Autodesk Inventor part; units mm, degrees
ref_plane "YZ Plane" through (0, 0, 0) normal (1, 0, 0) x (0, 1, 0)
ref_plane "XZ Plane" through (0, 0, 0) normal (0, 1, 0) x (-1, 0, 0)
ref_plane "XY Plane" through (0, 0, 0) normal (0, 0, 1) x (1, 0, 0)
sketch "Sketch1" plane through (0, 0, 0) normal (0, 0, 1) x (1, 0, 0)
  circle A0 centre (0, 0) radius 5
  arc A1 (-13, 15) -> (-15, 13) centre (-13, 13) ccw
  arc A2 (-15, -13) -> (-13, -15) centre (-13, -13) ccw
  arc A3 (13, -15) -> (15, -13) centre (13, -13) ccw
  arc A4 (15, 13) -> (13, 15) centre (13, 13) ccw
  arc A5 (-13, 14) -> (-14, 13) centre (-13, 13) ccw
  arc A6 (-14, -13) -> (-13, -14) centre (-13, -13) ccw
  arc A7 (13, -14) -> (14, -13) centre (13, -13) ccw
  arc A8 (14, 13) -> (13, 14) centre (13, 13) ccw
  line L0 (14, -14) -> (-14, 14) construction
  line L1 (-14, -14) -> (14, 14) construction
  line L2 (15, -15) -> (-15, 15) construction
  line L3 (-15, -15) -> (15, 15) construction
  line L4 (-13, 15) -> (-8, 15)
  line L5 (-8, 13) -> (-8, 8) construction
  line L6 (-9.4142, 8) -> (-13, 8)
  line L7 (-15, 8) -> (-15, 13)
  line L8 (-13, -15) -> (-8, -15)
  line L9 (-8, -13) -> (-8, -9.4142)
  line L10 (-9.4142, -8) -> (-13, -8)
  line L11 (-15, -8) -> (-15, -13)
  line L12 (13, -15) -> (8, -15)
  line L13 (8, -13) -> (8, -9.4142)
  line L14 (9.4142, -8) -> (13, -8)
  line L15 (15, -8) -> (15, -13)
  line L16 (13, 15) -> (8, 15)
  line L17 (8, 13) -> (8, 9.4142)
  line L18 (9.4142, 8) -> (13, 8)
  line L19 (15, 8) -> (15, 13)
  line L20 (-13, 9) -> (-10, 9)
  line L21 (-9, 10) -> (-9, 13)
  line L22 (-10, 14) -> (-13, 14)
  line L23 (-14, 13) -> (-14, 10)
  line L24 (13, 9) -> (10, 9)
  line L25 (9, 10) -> (9, 13)
  line L26 (10, 14) -> (13, 14)
  line L27 (14, 13) -> (14, 10)
  line L28 (13, -9) -> (10, -9)
  line L29 (9, -10) -> (9, -13)
  line L30 (10, -14) -> (13, -14)
  line L31 (14, -13) -> (14, -10)
  line L32 (-13, -9) -> (-10, -9)
  line L33 (-9, -10) -> (-9, -13)
  line L34 (-10, -14) -> (-13, -14)
  line L35 (-14, -13) -> (-14, -10)
  line L36 (-14, 13) -> (-14, 10)
  line L37 (-14, -10) -> (-14, -13)
  line L38 (-14, -13) -> (-14, -10)
  line L39 (-14, 10) -> (-14, 13)
  line L40 (13, -15) -> (5, -15)
  line L41 (-5, -15) -> (-13, -15)
  line L42 (13, -15) -> (5, -15) construction
  line L43 (0, -15) -> (-13, -15) construction
  line L44 (4, -13) -> (8, -13)
  line L45 (-8, -13) -> (-4, -13)
  line L46 (10, -9) -> (13, -9)
  line L47 (14, -10) -> (14, -13)
  line L48 (13, -14) -> (10, -14)
  line L49 (9, -13) -> (9, -10)
  line L50 (5, -14) -> (5, -15)
  line L51 (13, -14) -> (10, -14)
  line L52 (5, -14) -> (4, -14)
  line L53 (4, -14) -> (5, -14)
  line L54 (10, -14) -> (13, -14)
  line L55 (-4, -14) -> (-5, -14)
  line L56 (-10, -14) -> (-13, -14)
  line L57 (-13, -14) -> (-10, -14)
  line L58 (-5, -14) -> (-4, -14)
  line L59 (14, -13) -> (14, -10)
  line L60 (14, 10) -> (14, 13)
  line L61 (14, 13) -> (14, 10)
  line L62 (14, -10) -> (14, -13)
  line L63 (-5, -14) -> (-5, -15)
  line L64 (10, 14) -> (13, 14)
  line L65 (13, 14) -> (10, 14)
  line L66 (-10, 14) -> (-13, 14)
  line L67 (-13, 14) -> (-10, 14)
  line L68 (-5, 15) -> (-5, 14)
  line L69 (-13, 15) -> (-5, 15)
  line L70 (5, 15) -> (13, 15)
  line L71 (-15, 15) -> (-5, 15) construction
  line L72 (5, 15) -> (15, 15) construction
  line L73 (5, 15) -> (5, 14)
  line L74 (8, 13) -> (4, 13)
  line L75 (5, 14) -> (4, 14)
  line L76 (-5, 14) -> (-4, 14)
  line L77 (4, 14) -> (5, 14)
  line L78 (-4, 13) -> (-8, 13)
  line L79 (-4, 14) -> (-5, 14)
  line L80 (4, 13) -> (4, 14)
  line L81 (-4, 13) -> (-4, 14)
  line L82 (-4, -14) -> (-4, -13)
  line L83 (4, -14) -> (4, -13)
  line L84 (-8, 9.4142) -> (-4.1919, 5.6061)
  line L85 (8, 9.4142) -> (4.1919, 5.6061)
  line L86 (9.4142, 8) -> (5.6061, 4.1919)
  line L87 (5.6061, -4.1919) -> (9.4142, -8)
  line L88 (4.1919, -5.6061) -> (8, -9.4142)
  line L89 (-4.1919, -5.6061) -> (-8, -9.4142)
  line L90 (-5.6061, -4.1919) -> (-9.4142, -8)
  line L91 (-9.4142, 8) -> (-5.6061, 4.1919)
  arc A9 (4.1919, 5.6061) -> (-4.1919, 5.6061) centre (0, 0) ccw
  arc A10 (5.6061, -4.1919) -> (5.6061, 4.1919) centre (0, 0) ccw
  arc A11 (-5.6061, 4.1919) -> (-5.6061, -4.1919) centre (0, 0) ccw
  arc A12 (-4.1919, -5.6061) -> (4.1919, -5.6061) centre (0, 0) ccw
  line L92 (-8, 13) -> (-8, 9.4142)
  line L93 (-15, -13) -> (-15, -5) construction
  line L94 (-15, -13) -> (-15, -5)
  line L95 (-15, 5) -> (-15, 13)
  line L96 (15, -5) -> (15, -13) construction
  line L97 (15, 13) -> (15, 5)
  line L98 (15, -5) -> (15, -13)
  line L99 (-14, -4) -> (-14, -5)
  line L100 (14, -4) -> (14, -5)
  line L101 (14, 4) -> (14, 5)
  line L102 (-14, 4) -> (-14, 5)
  line L103 (-13, 8) -> (-13, 4)
  line L104 (13, 4) -> (13, 8)
  line L105 (13, -8) -> (13, -4)
  line L106 (-13, -4) -> (-13, -8)
  line L107 (-14, -5) -> (-15, -5)
  line L108 (15, -5) -> (14, -5)
  line L109 (15, 5) -> (14, 5)
  line L110 (-14, 5) -> (-15, 5)
  line L111 (13, 4) -> (14, 4)
  line L112 (-14, 4) -> (-13, 4)
  line L113 (-14, -4) -> (-13, -4)
  line L114 (13, -4) -> (14, -4)
  arc A13 (-13, -9) -> (-14, -10) centre (-13, -10) ccw
  arc A14 (-9, -10) -> (-10, -9) centre (-10, -10) ccw
  arc A15 (-10, -14) -> (-9, -13) centre (-10, -13) ccw
  arc A16 (10, -9) -> (9, -10) centre (10, -10) ccw
  arc A17 (9, -13) -> (10, -14) centre (10, -13) ccw
  arc A18 (14, -10) -> (13, -9) centre (13, -10) ccw
  arc A19 (10, 14) -> (9, 13) centre (10, 13) ccw
  arc A20 (9, 10) -> (10, 9) centre (10, 10) ccw
  arc A21 (13, 9) -> (14, 10) centre (13, 10) ccw
  arc A22 (-9, 13) -> (-10, 14) centre (-10, 13) ccw
  arc A23 (-10, 9) -> (-9, 10) centre (-10, 10) ccw
  arc A24 (-14, 10) -> (-13, 9) centre (-13, 10) ccw
  point P0 (15, -15)
  point P1 (-5.5858, -7)
  dimension "d0" = 30
  dimension "d1" = 30
  dimension "d2" = 10
  dimension "d4" = 2
  dimension "d11" = 28
  dimension "d12" = 7
  dimension "d13" = 7
  dimension "d15" = 1
  dimension "d16" = 1
  dimension "d17" = 1
  dimension "d18" = 1
  dimension "d19" = 5
  dimension "d23" = 30
  dimension "d27" = 1
  dimension "d30" = 3.5858
  dimension "d31" = 2
  dimension "d32" = 16
  dimension "d33" = 8
  dimension "d34" = 6
  dimension "d35" = 5.5858
extrude "Extrusion1" add sketch "Sketch1" along normal mid plane 318
properties part number "trail" material "Aluminum 6061"
Check sheet for the modelled part. Datum: model origin and axes. Units: mm. Give positions to 0.01 mm unless a question says otherwise; leave off trailing zeros. Write each loop counter-clockwise with the first axis right and the second up, starting at its lowest first coordinate (ties: lowest second). Pieces come first, ordered by that corner, then holes. Notation, with made-up numbers: (33, -29.75) -> (75, -29.75) arc R23 cw to (75, 0.25) -> close; hole circle Ø2 at (21.5, -25.5). An arc over 180 degrees is marked (long way). Use one line per item in the form item = value. Start each with the question number.
1. Mould release check, pull along Y, two halves, no side actions. Record for faces 1 (the flat face through (-15, -9, -2)), 2 (the flat face through (9, 15, -2)), 3 (the cylindrical face through (-7, 0, -2)): pulls with the +Y half, pulls with the -Y half, needs draft (parallel to the pull), parting line crosses it, or undercut.
2. Thickness scan on line 1 along X through (y, z) = (-12.5, -56); line 2 along Y through (x, z) = (0, -35); line 3 along Y through (x, z) = (-9.5, 15). Record the ranges inside material, lowest first. Write a range as from..to.
3. Section check A-A (x = 0). Record the cut outline in (y, z).
4. Section check C-C (z = -128.5). Count the separate pieces of the cut face and the enclosed holes in it, and give its area (3 significant figures).
5. Go/stop test with a flat-tipped pin: P1, Ø0.8, axis at y = -13.5, z = -67.5, coming from the +X side. Record where the tip stops, or that it passes through.
Conclusion:
q1.face_1 = needs draft
q1.face_2 = pulls with the +Y half
q1.face_3 = undercut
q2.line_1 = -15..-14, -9..-8, 8..9, 14..15
q2.line_2 = -7..-5, 5..7
q2.line_3 = -15..-13.87, -9.13..-8, 8..9.13, 13.87..15
q3.outline = (-7, -159) -> (-5, -159) -> (-5, 159) -> (-7, 159) -> close; (5, -159) -> (7, -159) -> (7, 159) -> (5, 159) -> close
q4.separate_pieces = 1
q4.enclosed_holes = 5
q4.area = 266 mm²
q5.P1 = 15
